The model under review builds one solid part; all positions refer to its coordinate system, in mm. A direction names the side the tool comes from. Round coordinates to 2 decimals unless told otherwise and drop trailing zeros. Write each loop counter-clockwise with the first axis right and the second up, starting at its lowest first coordinate (ties: lowest second). Pieces come first, ordered by that corner, then holes. Notation, with made-up numbers: (54, 44.5) - (75, 44.5) arc R23 ccw to (75, 67.5) - close; hole circle Ø10 at (-20.5, 87). An arc over 180 degrees is marked (long way). Return JSON: item names as keys, results as strings.
from build123d import *

# Parameters (mm, degrees)
F0_W     = 82.75
F0_H     = 82.75
F0_R     = 4.25
F0_R_2   = 31.75
F1_DEPTH = 6.5
F2_R     = 9.625
F3_R     = 34.875
F3_R_2   = 31.75
F4_DEPTH = 3.25


with BuildPart() as f1:
    # F0 (on Top) → F1 (new body)
    with BuildSketch(Plane.XY):
        Rectangle(F0_W, F0_H)
        with Locations((-31.75, -31.75)):
            Circle(F0_R, mode=Mode.SUBTRACT)
        with Locations((31.75, -31.75)):
            Circle(F0_R, mode=Mode.SUBTRACT)
        with Locations((-31.75, 31.75)):
            Circle(F0_R, mode=Mode.SUBTRACT)
        Circle(F0_R_2, mode=Mode.SUBTRACT)
        with Locations((31.75, 31.75)):
            Circle(F0_R, mode=Mode.SUBTRACT)
    extrude(amount=F1_DEPTH)

    # F2
    f2_edges = [f1.edges().sort_by_distance(p)[0] for p in [
        (-41.375, -41.375, 3.25),
        (-41.375, 41.375, 3.25),
        (41.375, 41.375, 3.25),
        (41.375, -41.375, 3.25),
    ]]
    fillet(f2_edges, radius=F2_R)

    # F3 (on face) → F4 (join)
    with BuildSketch(Plane.XY.offset(6.5)):
        Circle(F3_R)
        Circle(F3_R_2, mode=Mode.SUBTRACT)
    extrude(amount=F4_DEPTH)


solid = f1.part
(1) Add section A-A (y = 0). Write out the cut boundary in (x, z) (3 decimals).
Filled in:
{"outline": "(-41.375, 0) - (-31.75, 0) - (-31.75, 9.75) - (-34.875, 9.75) - (-34.875, 6.5) - (-41.375, 6.5) - close; (31.75, 0) - (41.375, 0) - (41.375, 6.5) - (34.875, 6.5) - (34.875, 9.75) - (31.75, 9.75) - close"}
(2) For faces 4 (the cylindrical face through (28.38, 29.16, 3.2)), 5 (the flat face through (36, 1, 6.5)), list the 3-axis set-ups (+Z, -Z, +X, -X, +Y, -Y) from which the entire face can be reached by the end or side of a thin tool; tool diameter is ignored.
Filled in:
{"face 4": "+Z, -Z", "face 5": "+Z"}
(3) Wall thickness on line 1 (Y direction, x = 32, z = 4.25); line 2 (Y direction, x = 33.5, z = 0.5); line 3 (Y direction, x = 0, z = 2) (3 decimals): over which ranges is each line inside the solid? List them lowest first.
Filled in:
{"line 1": "y = -41.37 to -35.99, -27.51 to 27.51, 35.99 to 41.37", "line 2": "y = -41.21 to -35.62, -27.88 to 27.88, 35.62 to 41.21", "line 3": "y = -41.375 to -31.75, 31.75 to 41.375"}
(4) Mouldability with a two-part tool opening along X and no side actions: class faces 1 (the flat face through (0, -41.375, 3)), 2 (the cylindrical face through (-35.996, -31.563, 3.204)), 3 (the flat face through (41.375, 0, 3)) as released by +X, released by -X, zero draft, split by the parting line, or undercut.
Filled in:
{"face 1": "zero draft", "face 2": "undercut", "face 3": "released by +X"}
(5) Add section D-D (y = -30). Write out the cut boundary in (x, z) (3 decimals), plus the area to 3 significant figures.
Filled in:
{"outline": "(-41.375, 0) - (-35.623, 0) - (-35.623, 6.5) - (-41.375, 6.5) - close; (-27.877, 0) - (-10.395, 0) - (-10.395, 9.75) - (-17.784, 9.75) - (-17.784, 6.5) - (-27.877, 6.5) - close; (10.395, 0) - (27.877, 0) - (27.877, 6.5) - (17.784, 6.5) - (17.784, 9.75) - (10.395, 9.75) - close; (35.623, 0) - (41.375, 0) - (41.375, 6.5) - (35.623, 6.5) - close", "area": "350 mm2"}
(6) Add section C-C (z = 5). Write out the cut boundary in (x, y) (3 decimals), plus the area to 3 significant figures.
Filled in:
{"outline": "(-41.375, -31.75) arc R9.625 ccw to (-31.75, -41.375) - (31.75, -41.375) arc R9.625 ccw to (41.375, -31.75) - (41.375, 31.75) arc R9.625 ccw to (31.75, 41.375) - (-31.75, 41.375) arc R9.625 ccw to (-41.375, 31.75) - close; hole circle Ø8.5 at (-31.75, -31.75); hole circle Ø8.5 at (-31.75, 31.75); hole circle Ø63.5 at (0, 0); hole circle Ø8.5 at (31.75, -31.75); hole circle Ø8.5 at (31.75, 31.75)", "area": "3,370 mm2"}
(7) Clearance check with a flat-ended pin moving along its axis: pin 1 Ø1 at (x, y) = (29.5, 27) entering from +Z. State where the tip first meets the part, or that it passes through.
Filled in:
{"pin 1": "stops at z = 6.5"}
